Design review of the part built by this model. Coordinates are the model's own, in mm. A direction names the side the tool comes from. Coordinates: 2 decimals unless noted, no trailing zeros. Write each loop counter-clockwise with the first axis right and the second up, starting at its lowest first coordinate (ties: lowest second). Pieces come first, ordered by that corner, then holes. Notation, with made-up numbers: M 6,4 L 23,4 A10 ccw 23,17 Z; hole C 23.5,26 d8. An arc over 180 degrees is marked long. Write each question's results on one line, items separated by ' | '. Start each with the question number.
```python
from build123d import *

# Parameters (mm, degrees)
SKETCH1_W           = 36
SKETCH1_H           = 17
BOSS_EXTRUDE1_DEPTH = 3
SKETCH15_W          = 36
SKETCH15_H          = 3
BOSS_EXTRUDE2_DEPTH = 14
FILLET2_R           = 2
FILLET3_R           = 4
SKETCH17_R          = 4
CUT_EXTRUDE1_DEPTH  = 18
SKETCH18_R          = 4
CUT_EXTRUDE2_DEPTH  = 18


with BuildPart() as part:
    # Sketch1 → Boss-Extrude1 (new body)
    with BuildSketch(Plane.XY):
        Rectangle(SKETCH1_W, SKETCH1_H)
    extrude(amount=BOSS_EXTRUDE1_DEPTH)

    # Sketch15 → Boss-Extrude2 (add)
    with BuildSketch(Plane.XY.offset(3)):
        with Locations((0, 7)):
            Rectangle(SKETCH15_W, SKETCH15_H)
    extrude(amount=BOSS_EXTRUDE2_DEPTH)

    # Fillet2
    fillet2_edges = [part.edges().sort_by_distance(p)[0] for p in [
        (0, 5.5, 3),
    ]]
    fillet(fillet2_edges, radius=FILLET2_R)

    # Fillet3
    fillet3_edges = [part.edges().sort_by_distance(p)[0] for p in [
        (0, 8.5, 0),
    ]]
    fillet(fillet3_edges, radius=FILLET3_R)

    # Sketch17 → Cut-Extrude1 (cut, through all)
    with BuildSketch(Plane.XZ.offset(8.5)):
        with Locations((10, 10)):
            Circle(SKETCH17_R)
    extrude(amount=-CUT_EXTRUDE1_DEPTH, mode=Mode.SUBTRACT)

    # Sketch18 → Cut-Extrude2 (cut, through all)
    with BuildSketch(Plane.XY.offset(17)):
        with Locations((-10, -1.5)):
            Circle(SKETCH18_R)
    extrude(amount=-CUT_EXTRUDE2_DEPTH, mode=Mode.SUBTRACT)


solid = part.part
```
Item 1: We need section C-C on z = 10. State the section outline as (x, y) points.
Item 2: We need section A-A on x = -9. State the section outline as (y, z) points.
Item 3: Wall thickness on L1, parallel to Y at x = -8, z = 5.5; L2, parallel to Z at x = 5, y = -4; L3, parallel to X at y = -5, z = 2.5: over which ranges is each line inside the solid? List them lowest first.
Item 4: Draft analysis for pull direction Y (two halves, no side actions). For faces 1 (the cylindrical face through (-13.996, -1.324, 1.521)), 2 (the flat face through (-18, 1.8, 2.7)), 3 (the flat face through (0, 5.5, 11)), state which applies: released by +Y, released by -Y, zero draft, split by the parting line, or undercut.
Item 5: Insertion check: pin 1 Ø3 at (x, z) = (-6, 13.5) entering from -Y; pin 2 Ø2 at (x, y) = (-13, -2) entering from +Z. Each pin has a flat end and moves straight along its axis. Give the tip position at first contact, or say it passes through.
Item 6: We need section D-D on x = 4. State the section outline as (y, z) points.
Item 7: For faces 4 (the flat face through (0, -2, 3)), 5 (the flat face through (0, 7, 17)), list the 3-axis set-ups (+Z, -Z, +X, -X, +Y, -Y) from which the entire face can be reached by the end or side of a thin tool; tool diameter is ignored.
Item 8: We need section B-B on y = 1. State the section outline as (x, z) points.
Answer:
1) outline: M -18,5.5 L 6,5.5 L 6,8.5 L -18,8.5 Z; M 14,5.5 L 18,5.5 L 18,8.5 L 14,8.5 Z
2) outline: M -8.5,0 L -5.37,0 L -5.37,3 L -8.5,3 Z; M 2.37,0 L 4.5,0 A4 ccw 8.5,4 L 8.5,17 L 5.5,17 L 5.5,5 A2 cw 3.5,3 L 2.37,3 Z
3) L1: y = 5.5 to 8.5 | L2: z = 0 to 3 | L3: x = -18 to -11.94, -8.06 to 18
4) face 1: undercut | face 2: zero draft | face 3: released by -Y
5) pin 1: stops at y = 5.5 | pin 2: stops at z = 3
6) outline: M -8.5,0 L 4.5,0 A4 ccw 8.5,4 L 8.5,17 L 5.5,17 L 5.5,5 A2 cw 3.5,3 L -8.5,3 Z
7) face 4: +Z, +X, -X, -Y | face 5: +Z, +X, -X, +Y, -Y
8) outline: M -18,0 L -13.12,0 L -13.12,3 L -18,3 Z; M -6.88,0 L 18,0 L 18,3 L -6.88,3 Z
